```python
from build123d import *

# Parameters (mm, degrees)
EXTRUDE1_DEPTH      = 2.25
EXTRUDE2_DEPTH      = 12
CHAMFER1_SIZE       = 5.1
CHAMFER1_SIZE2      = 6.76792859
SKETCH6_W           = 60
SKETCH6_H           = 26.1
CUT_EXTRUDE1_DEPTH  = 8.4
SKETCH9_W           = 10
SKETCH9_H           = 40
CUT_EXTRUDE3_DEPTH  = 37.363978582
SKETCH10_W          = 44
SKETCH10_H          = 20
CUT_EXTRUDE4_DEPTH  = 3.1
CUT_EXTRUDE8_DEPTH  = 13
SKETCH16_R          = 1.525
CUT_EXTRUDE9_DEPTH  = 34.212384738
SKETCH17_R          = 2.275
CUT_EXTRUDE10_DEPTH = 34.212384908
EXTRUDE4_START      = 0.3
SKETCH18_R          = 3.05
SKETCH18_R_2        = 2.275
EXTRUDE4_DEPTH      = 0.3
FILLET1_R           = 1.2


with BuildPart() as part:
    # Sketch1 → Extrude1 (new body)
    with BuildSketch(Plane.XY):
        with BuildLine():
            ThreePointArc((-22.224984725, -0.026057486), (0.013028745, -22.224996181), (22.225, 0))
            ThreePointArc((22.225, 0), (-0.013028745, 22.224996181), (-22.224984725, -0.026057486))
        make_face()
    extrude(amount=EXTRUDE1_DEPTH)

    # Sketch2 → Extrude2 (add)
    with BuildSketch(Plane.XY.offset(2.25)):
        with BuildLine():
            ThreePointArc((-23.999872331, -0.078282234), (0.113586787, -23.999731208), (23.999538151, 0.148891095))
            ThreePointArc((23.999538151, 0.148891095), (-0.113586787, 23.999731208), (-23.999872331, -0.078282234))
        make_face()
    extrude(amount=EXTRUDE2_DEPTH)

    # Chamfer1
    chamfer1_edges = [part.edges().sort_by_distance(p)[0] for p in [
        (-23.999538151, -0.148891095, 14.25),
    ]]
    chamfer1_side = [part.faces().sort_by_distance(p)[0] for p in [
        (0, 0, 14.25),
    ]]
    chamfer(chamfer1_edges, length=CHAMFER1_SIZE, length2=CHAMFER1_SIZE2, reference=chamfer1_side[0])

    # Sketch6 → Cut-Extrude1 (cut)
    with BuildSketch(Plane(origin=(0, 0, 0), x_dir=(-1, 0, 0), z_dir=(0, 0, -1))):
        Rectangle(SKETCH6_W, SKETCH6_H)
    extrude(amount=-CUT_EXTRUDE1_DEPTH, mode=Mode.SUBTRACT)

    # Sketch9 → Cut-Extrude3 (cut, through all)
    with BuildSketch(Plane(origin=(0, 0, 0), x_dir=(-1, 0, 0), z_dir=(0, 0, -1))):
        with Locations((-23, 0)):
            Rectangle(SKETCH9_W, SKETCH9_H)
        with Locations((23, 0)):
            Rectangle(SKETCH9_W, SKETCH9_H)
    extrude(amount=-CUT_EXTRUDE3_DEPTH, mode=Mode.SUBTRACT)

    # Sketch10 → Cut-Extrude4 (cut)
    with BuildSketch(Plane(origin=(0, 0, 8.4), x_dir=(-1, 0, 0), z_dir=(0, 0, -1))):
        Rectangle(SKETCH10_W, SKETCH10_H)
    extrude(amount=-CUT_EXTRUDE4_DEPTH, mode=Mode.SUBTRACT)

    # Sketch15 → Cut-Extrude8 (cut)
    with BuildSketch(Plane(origin=(0, 0, 0), x_dir=(-1, 0, 0), z_dir=(0, 0, -1))):
        with BuildLine():
            Line((4, -13), (4, 13))
            ThreePointArc((4, 13), (0, 17), (-4, 13))
            Line((-4, 13), (-4, -13))
            ThreePointArc((-4, -13), (0, -17), (4, -13))
        make_face()
    extrude(amount=-CUT_EXTRUDE8_DEPTH, mode=Mode.SUBTRACT)

    # Sketch16 → Cut-Extrude9 (cut, through all)
    with BuildSketch(Plane(origin=(0, 0, 0), x_dir=(-1, 0, 0), z_dir=(0, 0, -1))):
        with Locations((-10, -16.5)):
            Circle(SKETCH16_R)
        with Locations(Location((10, -16.5, 0), (0, 0, 48.382100449))):
            Circle(SKETCH16_R)
        with Locations((10, 16.5)):
            Circle(SKETCH16_R)
        with Locations(Location((-10, 16.5, 0), (0, 0, 14.054705204))):
            Circle(SKETCH16_R)
    extrude(amount=-CUT_EXTRUDE9_DEPTH, mode=Mode.SUBTRACT)

    # Sketch17 → Cut-Extrude10 (cut, through all)
    with BuildSketch(Plane.XY.offset(14.25)):
        Circle(SKETCH17_R)
    extrude(amount=-CUT_EXTRUDE10_DEPTH, mode=Mode.SUBTRACT)

    # Sketch18 → Extrude4 (add)
    with BuildSketch(Plane.XY.offset(14.25).offset(EXTRUDE4_START)):
        with Locations(Location((0, 0, 0), (0, 0, 180))):
            Circle(SKETCH18_R)
        Circle(SKETCH18_R_2, mode=Mode.SUBTRACT)
    extrude(amount=-EXTRUDE4_DEPTH)

    # Fillet1
    fillet1_edges = [part.edges().sort_by_distance(p)[0] for p in [
        (-2.275, 0, 13),
    ]]
    fillet(fillet1_edges, radius=FILLET1_R)


solid = part.part
```
Build history of the part. All positions in model axes, mm. A direction names the side the tool comes from. Round coordinates to 2 decimals unless told otherwise and drop trailing zeros. Write each loop counter-clockwise with the first axis right and the second up, starting at its lowest first coordinate (ties: lowest second). Pieces come first, ordered by that corner, then holes. Notation, with made-up numbers: (25.25, 76) -> (37.25, 76) arc R15 ccw to (37.25, 104) -> close; hole circle Ø11 at (35, 85.25). An arc over 180 degrees is marked (long way). Put each result on its own line as item: value.
Item 1: Two-plate mould, pull along X, no slides. Class faces 1 (the face through (0.36, 20.35, 12.32)), 2 (the face through (0, -4, 13)), 3 (the face through (0, -18, 0)): pulls with the +X half, pulls with the -X half, needs draft (parallel to the pull), parting line crosses it, or undercut.
Here are the results:
face 1: parting line crosses it
face 2: undercut
face 3: needs draft
Item 2: Wall check: probe 1 along X at (y, z) = (16.5, 3.5) (1 decimal); probe 2 along X at (y, z) = (-16.5, 8) (1 decimal); probe 3 along Y at (x, z) = (11, 5.25). Give the ranges that are in metal, low to high. Write a range as from..to.
Here are the results:
probe 1: x = -17.4..-11.5, -8.5..-1.9, 1.9..8.5, 11.5..17.4
probe 2: x = -16.9..-11.5, -8.5..-1.9, 1.9..8.5, 11.5..16.9
probe 3: y = -21.33..-17.65, -15.35..-13.05, 13.05..15.35, 17.65..21.33
Item 3: Tool access for faces 4 (the face through (0, -17, 6)), 5 (the face through (0, -23, 2.25)), 6 (the face through (-11, -12, 8.4)): list every direction of +Z, -Z, +X, -X, +Y, -Y with a clear straight run to the whole face (end or side of a thin tool).
Here are the results:
face 4: -Z
face 5: -Z, -Y
face 6: -Z, +X, -X
Item 4: Flat gauge pins, fed straight in: P1, Ø11, axis at x = -6, y = -8.5, coming from the +Z side; P2, Ø4, axis at x = 12, z = 9, coming from the -Y side; P3, Ø4, axis at x = 4.5, z = 12, coming from the -Y side; P4, Ø1.8, axis at x = -10, y = 16.5, coming from the +Z side. Where does each tip first touch, or does it go through?
Here are the results:
P1: stops at z = 14.25
P2: stops at y = -21.48
P3: stops at y = -21.69
P4: passes through
Item 5: Slice it at A-A, the plane x = 0. Give the cut face in (y, z) (3 decimals), plus the area to 3 significant figures.
Here are the results:
outline: (-24, 2.25) -> (-22.225, 2.25) -> (-22.225, 0) -> (-17, 0) -> (-17, 13) -> (-3.475, 13) arc R1.2 ccw to (-2.275, 14.2) -> (-2.275, 14.55) -> (-3.05, 14.55) -> (-3.05, 14.25) -> (-18.9, 14.25) -> (-24, 7.482) -> close; (2.275, 14.2) arc R1.2 ccw to (3.475, 13) -> (17, 13) -> (17, 0) -> (22.225, 0) -> (22.225, 2.25) -> (24, 2.25) -> (24, 7.482) -> (18.9, 14.25) -> (3.05, 14.25) -> (3.05, 14.55) -> (2.275, 14.55) -> close
area: 194 mm^2
Item 6: Slice it at C-C, the plane z = 3. Count the separate pieces of the cut face and the enclosed holes in it, plus the area to 3 significant figures.
Here are the results:
separate pieces: 2
enclosed holes: 4
area: 530 mm^2
